```python
from build123d import *

# Parameters (mm, degrees)
CROQUIS1_R              = 1.6
SALIENTE_EXTRUIR1_DEPTH = 3
REDONDEO1_R             = 3


with BuildPart() as part:
    # Croquis1 → Saliente-Extruir1 (new body)
    with BuildSketch(Plane(origin=(0, 0, 0), x_dir=(1, 0, 0), z_dir=(0, 1, 0))):
        Polygon((-5, 23.5), (-5, -23.5), (20.527864045, -36.263932023), (25, -27.319660113), (5, -17.319660113), (5, 17.319660113), (25, 27.319660113), (20.527864045, 36.263932023), align=None)
        with Locations(Location((0, 20, 0), (0, 0, 270))):
            Circle(CROQUIS1_R, mode=Mode.SUBTRACT)
        with Locations(Location((0, -20, 0), (0, 0, 270))):
            Circle(CROQUIS1_R, mode=Mode.SUBTRACT)
        with Locations(Location((20, 30, 0), (0, 0, 270))):
            Circle(CROQUIS1_R, mode=Mode.SUBTRACT)
        with Locations(Location((20, -30, 0), (0, 0, 270))):
            Circle(CROQUIS1_R, mode=Mode.SUBTRACT)
    extrude(amount=SALIENTE_EXTRUIR1_DEPTH)

    # Redondeo1
    redondeo1_edges = [part.edges().sort_by_distance(p)[0] for p in [
        (25, 1.5, 27.319660113),
        (20.527864045, 1.5, 36.263932023),
        (-5, 1.5, 23.5),
        (-5, 1.5, -23.5),
        (20.527864045, 1.5, -36.263932023),
        (25, 1.5, -27.319660113),
        (5, 1.5, -17.319660113),
        (5, 1.5, 17.319660113),
    ]]
    fillet(redondeo1_edges, radius=REDONDEO1_R)


solid = part.part
```
Could you check a few things on this model? Use its own coordinates, in mm. A direction names the side the tool comes from. Coordinates: 2 decimals unless noted, no trailing zeros. Write each loop counter-clockwise with the first axis right and the second up, starting at its lowest first coordinate (ties: lowest second). Pieces come first, ordered by that corner, then holes. Notation, with made-up numbers: (14.25, 30) -> (25.25, 30) arc R18 cw to (25.25, 43) -> close; hole circle Ø9 at (-12.5, 85). An arc over 180 degrees is marked (long way). Return JSON: item names as keys, results as strings.
(1) Imagine slicing it at C-C, the plane y = 0.5. Please give me the cut outline in (x, z).
Numbers:
{"outline": "(-5, -21.65) arc R3 ccw to (-3.34, -24.33) -> (17.84, -34.92) arc R3 ccw to (21.87, -33.58) -> (23.66, -30) arc R3 ccw to (22.32, -25.98) -> (6.66, -18.15) arc R3 cw to (5, -15.47) -> (5, 15.47) arc R3 cw to (6.66, 18.15) -> (22.32, 25.98) arc R3 ccw to (23.66, 30) -> (21.87, 33.58) arc R3 ccw to (17.84, 34.92) -> (-3.34, 24.33) arc R3 ccw to (-5, 21.65) -> close; hole circle Ø3.2 at (0, -20); hole circle Ø3.2 at (0, 20); hole circle Ø3.2 at (20, -30); hole circle Ø3.2 at (20, 30)"}
(2) I need wall thicknesses on L1, parallel to Z at x = 20.25, y = 0.25; L2, parallel to X at y = 1, z = 20; L3, parallel to Z at x = 8, y = 0.5. Which ranges of each line are inside material? Lowest first, please.
Numbers:
{"L1": "z = -35.04 to -31.58, -28.42 to -24.94, 24.94 to 28.42, 31.58 to 35.04", "L2": "x = -5 to -1.6, 1.6 to 10.36", "L3": "z = -30 to -18.82, 18.82 to 30"}
(3) We'd pull the mould along X, two halves only. Please class faces 3 (the cylindrical face through (-4.564, 1.521, -23.203)), 4 (the cylindrical face through (21.08, 1.48, -31.18)), 5 (the flat face through (22.776, 1.479, -31.767)): +X half, -X half, draft (parallel to the pull), parting line (faces both ways), or undercut.
Numbers:
{"face 3": "-X half", "face 4": "undercut", "face 5": "+X half"}
(4) Imagine slicing it at A-A, the plane x = 20. Please give me the cut outline in (y, z), then the cut area to 3 significant figures.
Numbers:
{"outline": "(0, -35.13) -> (3, -35.13) -> (3, -31.6) -> (0, -31.6) -> close; (0, -28.4) -> (3, -28.4) -> (3, -24.82) -> (0, -24.82) -> close; (0, 24.82) -> (3, 24.82) -> (3, 28.4) -> (0, 28.4) -> close; (0, 31.6) -> (3, 31.6) -> (3, 35.13) -> (0, 35.13) -> close", "area": "42.6 mm2"}
(5) Which directions (+Z, -Z, +X, -X, +Y, -Y) give clear straight access to the entire face, cutting with the end or side of a thin tool? Please do faces 1 (the cylindrical face through (20.104, 1.521, 35.095)), 2 (the cylindrical face through (5.46, 1.52, 17.06)).
Numbers:
{"face 1": "+Z, +Y, -Y", "face 2": "+X, +Y, -Y"}
(6) Imagine slicing it at B-B, the plane z = -20. Please give me the cut outline in (x, y), then the cut area to 3 significant figures.
Numbers:
{"outline": "(-5, 0) -> (-1.6, 0) -> (-1.6, 3) -> (-5, 3) -> close; (1.6, 0) -> (10.36, 0) -> (10.36, 3) -> (1.6, 3) -> close", "area": "36.5 mm2"}
(7) I'm going to push a flat-ended pin straight in: pin 1 (1.5 mm diameter, centred on y = 2, z = 7, fed in from +X). Where does the tip first touch, or does it pass through?
Numbers:
{"pin 1": "stops at x = 5"}
(8) Imagine slicing it at D-D, the plane x = 14. Please give me the cut outline in (y, z), then the cut area to 3 significant figures.
Numbers:
{"outline": "(0, -33) -> (3, -33) -> (3, -21.82) -> (0, -21.82) -> close; (0, 21.82) -> (3, 21.82) -> (3, 33) -> (0, 33) -> close", "area": "67.1 mm2"}
